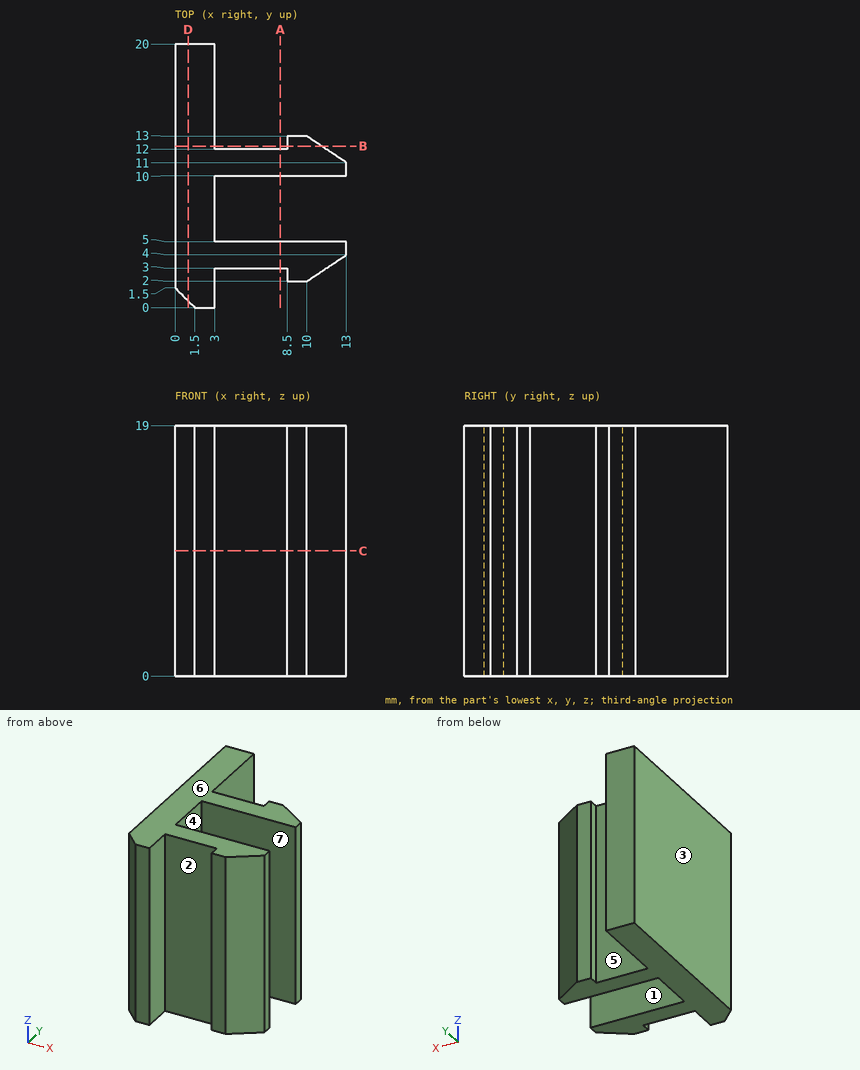
Geometry: see drawing. Coordinates: mm, zero at the bounding-box minimum. A direction names the side the tool comes from. Coordinates: 2 decimals unless noted, no trailing zeros. Loops run counter-clockwise (first coordinate to the right, second up) from the corner with the lowest first, then second, coordinate; pieces in that order, holes last. Notation, with made-up numbers: M -20.5,18 L 18.5,18 A13 ccw 18.5,38 Z; hole C 19,10.5 d6. An arc over 180 degrees is marked long. Answer in a Markdown table with one row per item.
Q1. Section C-C on z = 9.5. Return the cut outline in (x, y), plus the area to 3 significant figures.
Answers below:
| item | result |
|---|---|
| outline | M 0,1.5 L 1.5,0 L 3,0 L 3,3 L 8.5,3 L 8.5,2 L 10,2 L 13,4 L 13,5 L 3,5 L 3,10 L 13,10 L 13,11 L 10,13 L 8.5,13 L 8.5,12 L 3,12 L 3,20 L 0,20 Z |
| area | 102 mm^2 |
Q2. Set-up query: the marked faces 1, 2 and 3. Return all of +Z, -Z, +X, -X, +Y, -Y with unobstructed straight access to the full face (end or side cutting, diameter ignored); none if empty.
Answers below:
| item | result |
|---|---|
| face 1 | +Z, -Z, +X |
| face 2 | +Z, -Z, -Y |
| face 3 | +Z, -Z, -X, +Y, -Y |
Q3. Section B-B on y = 12.25. Return the cut outline in (x, z) (3 decimals).
Answers below:
| item | result |
|---|---|
| outline | M 0,0 L 3,0 L 3,19 L 0,19 Z; M 8.5,0 L 11.125,0 L 11.125,19 L 8.5,19 Z |
Q4. Section D-D on x = 1. Return the cut outline in (y, z).
Answers below:
| item | result |
|---|---|
| outline | M 0.5,0 L 20,0 L 20,19 L 0.5,19 Z |
Q5. First-contact query: pin 1 (0.9 mm diameter, centred on y = 1, z = 14, fed in from +X); pin 2 (1.6 mm diameter, centred on x = 5.5, z = 8, fed in from -Y); pin 3 (1.6 mm diameter, centred on x = 4.5, z = 8, fed in from +Y). Flat tips, straight axial feed; report the tip coordinate or a pass-through.
Answers below:
| item | result |
|---|---|
| pin 1 | stops at x = 3 |
| pin 2 | stops at y = 3 |
| pin 3 | stops at y = 12 |
Q6. Ray query, probe 1 along Y at (x, z) = (9.5, 17.75); probe 2 along Y at (x, z) = (4.25, 11); probe 3 along X at (y, z) = (1.75, 3). Return the intervals inside material, ascending. Write a range as from..to.
Answers below:
| item | result |
|---|---|
| probe 1 | y = 2..5, 10..13 |
| probe 2 | y = 3..5, 10..12 |
| probe 3 | x = 0..3 |
Q7. Section A-A on x = 8. Return the cut outline in (y, z), plus the area to 3 significant figures.
Answers below:
| item | result |
|---|---|
| outline | M 3,0 L 5,0 L 5,19 L 3,19 Z; M 10,0 L 12,0 L 12,19 L 10,19 Z |
| area | 76.0 mm^2 |
Q8. Draft query along Y for the marked faces 4, 5, 6 and 7. Return one class per face: pulls with the +Y half, pulls with the -Y half, needs draft (parallel to the pull), parting line crosses it, or undercut.
Answers below:
| item | result |
|---|---|
| face 4 | undercut |
| face 5 | pulls with the +Y half |
| face 6 | needs draft |
| face 7 | undercut |
